from build123d import *

# Parameters (mm, degrees)
SALIENTE_EXTRUIR1_DEPTH = 5
CROQUIS2_R              = 17.2
CORTAR_EXTRUIR1_DEPTH   = 5
CROQUIS3_R              = 22.75
CORTAR_EXTRUIR2_DEPTH   = 2


with BuildPart() as part:
    # Croquis1 → Saliente-Extruir1 (new body)
    with BuildSketch(Plane.XY):
        Polygon((-100, -100), (-100, -20), (-105, -20), (-105, 20), (-100, 20), (-100, 100), (-20, 100), (-20, 95), (20, 95), (20, 100), (100, 100), (100, 20), (105, 20), (105, -20), (100, -20), (100, -100), (20, -100), (20, -95), (-20, -95), (-20, -100), align=None)
    extrude(amount=SALIENTE_EXTRUIR1_DEPTH)

    # Croquis2 → Cortar-Extruir1 (cut)
    with BuildSketch(Plane.XY.offset(5)):
        with Locations((-35, 50)):
            Circle(CROQUIS2_R)
    extrude(amount=-CORTAR_EXTRUIR1_DEPTH, mode=Mode.SUBTRACT)

    # Croquis3 → Cortar-Extruir2 (cut)
    with BuildSketch(Plane.XY.offset(5)):
        with Locations((-35, 50)):
            Circle(CROQUIS3_R)
    extrude(amount=-CORTAR_EXTRUIR2_DEPTH, mode=Mode.SUBTRACT)


solid = part.part
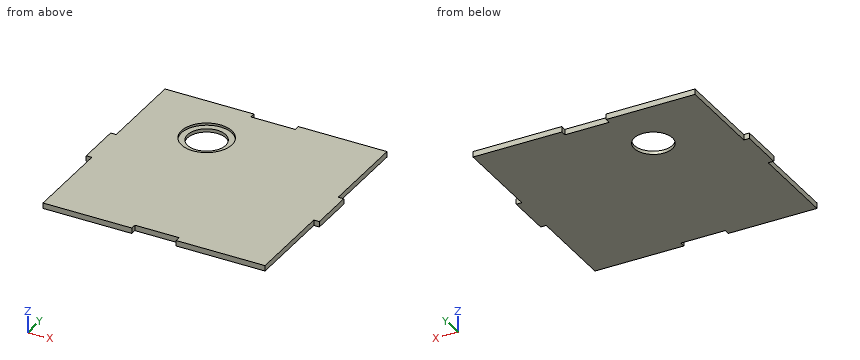
Part model, mm, in its own coordinate system. Coordinates: 2 decimals unless noted, no trailing zeros. Order: outer loops, then holes, each group sorted by start corner. A loop starts at its lowest first (then second) coordinate and runs counter-clockwise, first axis right, second up. Notation, with made-up numbers: M 84,76 L 94,76 A16 ccw 94,92 Z; hole C -22.5,70 d1. An arc over 180 degrees is marked long. Use a Markdown table: item, result.
(1) Cut at B-B on x = -35. Write the cut outline in (y, z).
A:
| item | result |
|---|---|
| outline | M -100,0 L 32.8,0 L 32.8,3 L 27.25,3 L 27.25,5 L -100,5 Z; M 67.2,0 L 100,0 L 100,5 L 72.75,5 L 72.75,3 L 67.2,3 Z |
(2) Cut at A-A on z = 1.4. Write the cut outline in (x, y).
A:
| item | result |
|---|---|
| outline | M -105,-20 L -100,-20 L -100,-100 L -20,-100 L -20,-95 L 20,-95 L 20,-100 L 100,-100 L 100,-20 L 105,-20 L 105,20 L 100,20 L 100,100 L 20,100 L 20,95 L -20,95 L -20,100 L -100,100 L -100,20 L -105,20 Z; hole C -35,50 d34.4 |
(3) Probe L1, parallel to X at y = 49.5, z = 0.5; L2, parallel to Y at x = -35, z = 1.05; L3, parallel to X at y = -45, z = 0.95. List the from-to ranges inside material, lowest first.
A:
| item | result |
|---|---|
| L1 | x = -100 to -52.19, -17.81 to 100 |
| L2 | y = -100 to 32.8, 67.2 to 100 |
| L3 | x = -100 to 100 |
(4) Cut at D-D on y = -58. Write the cut outline in (x, z).
A:
| item | result |
|---|---|
| outline | M -100,0 L 100,0 L 100,5 L -100,5 Z |
(5) Cut at C-C on y = 50. Write the cut outline in (x, z), then the cut area to 3 significant figures.
A:
| item | result |
|---|---|
| outline | M -100,0 L -52.2,0 L -52.2,3 L -57.75,3 L -57.75,5 L -100,5 Z; M -17.8,0 L 100,0 L 100,5 L -12.25,5 L -12.25,3 L -17.8,3 Z |
| area | 806 mm^2 |
(6) Flat gauge pins, fed straight in: pin 1 (2.5 mm diameter, centred on y = 78, z = 2, fed in from -X); pin 2 (1.5 mm diameter, centred on x = -102, z = 3.5, fed in from -Y); pin 3 (1.5 mm diameter, centred on x = -4, z = 1, fed in from -Y). Where does each tip first touch, or does it go through?
A:
| item | result |
|---|---|
| pin 1 | stops at x = -100 |
| pin 2 | stops at y = -20 |
| pin 3 | stops at y = -95 |
